Input: part model. Units: mm. Frame: model coordinates. A direction names the side the tool comes from. Coordinates: 2 decimals unless noted, no trailing zeros. Order: outer loops, then holes, each group sorted by start corner. A loop starts at its lowest first (then second) coordinate and runs counter-clockwise, first axis right, second up. Notation, with made-up numbers: M -28.75,32 L 20.25,32 A12 cw 20.25,54 Z; hole C 64,54 d4. An arc over 180 degrees is marked long. One line per item, written item: value.
```python
from build123d import *

# Parameters (mm, degrees)
BOSS_EXTRUDE1_DEPTH = 12.7
CUT_EXTRUDE2_DEPTH  = 199.932436772
CUT_EXTRUDE1_DEPTH  = 104.050150898
CUT_EXTRUDE3_DEPTH  = 63.5
CHAMFER1_SIZE       = 1.5875
FILLET1_R           = 0.762
FILLET2_R           = 1.27
CUT_EXTRUDE4_DEPTH  = 100.247182118


# Some blends are built 0.0001 mm under size
with BuildPart() as part:
    # Sketch1 → Boss-Extrude1 (new body)
    with BuildSketch(Plane(origin=(0, 0, 0), x_dir=(1, 0, 0), z_dir=(0, 1, 0))):
        with BuildLine():
            Line((-99.06, -12.7), (99.06, -12.7))
            Line((99.06, -12.7), (99.06, -11.1125))
            Line((99.06, -11.1125), (80.01, -11.1125))
            ThreePointArc((80.01, -11.1125), (75.519871939, -9.252628061), (73.66, -4.7625))
            Line((73.66, -4.7625), (73.66, 4.7625))
            ThreePointArc((73.66, 4.7625), (75.519871939, 9.252628061), (80.01, 11.1125))
            Line((80.01, 11.1125), (99.06, 11.1125))
            Line((99.06, 11.1125), (99.06, 12.7))
            Line((99.06, 12.7), (-99.06, 12.7))
            Line((-99.06, 12.7), (-99.06, 11.1125))
            Line((-99.06, 11.1125), (-80.01, 11.1125))
            ThreePointArc((-80.01, 11.1125), (-75.519871939, 9.252628061), (-73.66, 4.7625))
            Line((-73.66, 4.7625), (-73.66, -4.7625))
            ThreePointArc((-73.66, -4.7625), (-75.519871939, -9.252628061), (-80.01, -11.1125))
            Line((-80.01, -11.1125), (-99.06, -11.1125))
            Line((-99.06, -11.1125), (-99.06, -12.7))
        make_face()
    extrude(amount=BOSS_EXTRUDE1_DEPTH)

    # Sketch3 → Cut-Extrude2 (cut, through all)
    with BuildSketch(Plane.ZY.offset(99.06)):
        Polygon((11.1125, 12.7), (4.7625, 12.7), (-4.7625, 12.7), (-11.1125, 12.7), (-9.525, 6.35), (9.525, 6.35), align=None)
    extrude(amount=-CUT_EXTRUDE2_DEPTH, mode=Mode.SUBTRACT)

    # Sketch2 → Cut-Extrude1 (cut, through all)
    with BuildSketch(Plane.XY.offset(12.7)):
        Polygon((73.66, 12.7), (-73.66, 12.7), (-67.31, 6.35), (67.31, 6.35), align=None)
        with BuildLine():
            Line((97.263948776, 4.553948776), (92.71, 0))
            Line((92.71, 0), (99.06, 0))
            Line((99.06, 0), (99.06, 12.7))
            Line((99.06, 12.7), (92.71, 12.7))
            Line((92.71, 12.7), (97.263948776, 8.146051224))
            ThreePointArc((97.263948776, 8.146051224), (98.007897552, 6.35), (97.263948776, 4.553948776))
        make_face()
        with BuildLine():
            ThreePointArc((-97.263948776, 4.553948776), (-98.007897552, 6.35), (-97.263948776, 8.146051224))
            Line((-97.263948776, 8.146051224), (-92.71, 12.7))
            Line((-92.71, 12.7), (-99.06, 12.7))
            Line((-99.06, 12.7), (-99.06, 0))
            Line((-99.06, 0), (-92.71, 0))
            Line((-92.71, 0), (-97.263948776, 4.553948776))
        make_face()
    extrude(amount=-CUT_EXTRUDE1_DEPTH, mode=Mode.SUBTRACT)

    # Sketch4 → Revolve1 (revolve)
    with BuildSketch(Plane.ZY.offset(90.17)):
        with BuildLine():
            Line((12.7, 6.35), (12.7, 11.43))
            ThreePointArc((12.7, 11.43), (13.881381744, 9.01113492), (14.2875, 6.35))
            Line((14.2875, 6.35), (12.7, 6.35))
        make_face()
    revolve1 = revolve(axis=Axis((-90.17, 6.35, 0), (0, 0, 1)))

    # Mirror1: Revolve1 across plane
    add(revolve1.mirror(Plane.XY))

    # Sketch5 → Revolve2 (revolve)
    with BuildSketch(Plane(origin=(90.17, 0, 0), x_dir=(0, 0, -1), z_dir=(1, 0, 0))):
        with BuildLine():
            Line((11.1125, 6.35), (11.1125, 11.43))
            ThreePointArc((11.1125, 11.43), (9.931118256, 9.01113492), (9.525, 6.35))
            Line((9.525, 6.35), (11.1125, 6.35))
        make_face()
    revolve2 = revolve(axis=Axis((90.17, 6.35, 0), (0, 0, -1)))

    # Mirror2: Revolve2 across plane
    add(revolve2.mirror(Plane.XY))

    # Sketch6 → Cut-Extrude3 (cut, symmetric)
    with BuildSketch(Plane(origin=(0, 0, 0), x_dir=(0, 0, -1), z_dir=(1, 0, 0))):
        Polygon((-12.7, 0), (-11.1125, 0), (-12.7, 1.5875), align=None)
        Polygon((11.1125, 0), (12.7, 1.5875), (12.7, 0), align=None)
    extrude(amount=CUT_EXTRUDE3_DEPTH, both=True, mode=Mode.SUBTRACT)

    # Chamfer1
    chamfer1_edges = [part.edges().sort_by_distance(p)[0] for p in [
        (63.5, 0, 11.90625),
        (63.5, 0, -11.90625),
        (-63.5, 0, -11.90625),
        (-63.5, 0, 11.90625),
    ]]
    chamfer(chamfer1_edges, length=CHAMFER1_SIZE - 0.0001)  # a hair under: the kernel refuses the full size

    # Fillet1
    fillet1_edges = [part.edges().sort_by_distance(p)[0] for p in [
        (-98.007897552, 6.35, 12.7),
        (-92.71, 12.7, -11.90625),
        (-94.986974388, 10.423025612, -11.1125),
        (-94.986974388, 10.423025612, -12.7),
        (-94.986974388, 10.423025612, 11.1125),
        (-92.71, 12.7, 11.90625),
        (-94.986974388, 2.276974388, 12.7),
        (-98.007897552, 6.35, -11.1125),
        (-98.007897552, 6.35, 11.1125),
        (-94.986974388, 2.276974388, -11.1125),
        (-94.986974388, 2.276974388, 11.1125),
        (-98.007897552, 6.35, -12.7),
        (-94.986974388, 2.276974388, -12.7),
        (-94.986974388, 10.423025612, 12.7),
        (98.007897552, 6.35, 12.7),
        (92.71, 12.7, 11.90625),
        (92.71, 12.7, -11.90625),
        (94.986974388, 10.423025612, 12.7),
        (94.986974388, 2.276974388, 11.1125),
        (94.986974388, 2.276974388, -11.1125),
        (94.986974388, 2.276974388, -12.7),
        (98.007897552, 6.35, 11.1125),
        (94.986974388, 10.423025612, 11.1125),
        (94.986974388, 10.423025612, -11.1125),
        (98.007897552, 6.35, -12.7),
        (94.986974388, 10.423025612, -12.7),
        (94.986974388, 2.276974388, 12.7),
        (98.007897552, 6.35, -11.1125),
    ]]
    fillet(fillet1_edges, radius=FILLET1_R)

    # Fillet2
    # the kernel refuses this fillet: 1.27 mm, written as the material it takes off along each edge
    with BuildSketch(Plane(origin=(-75.90506403, 14.94506403, -12.7), x_dir=(-0.7071067811865446, -0.7071067811865505, 0), z_dir=(0.7071067811865506, -0.7071067811865446, 0))) as fillet2_piece_1_section:
        with BuildLine():
            CenterArc((FILLET2_R, -FILLET2_R), FILLET2_R, 90, 90)
            Line((0, -FILLET2_R), (0, 0))
            Line((0, 0), (FILLET2_R, 0))
        make_face()
    fillet2_piece_1 = extrude(amount=15.330256121, mode=Mode.PRIVATE)
    fillet2_piece_1 = split(fillet2_piece_1, bisect_by=Plane(origin=(-71.905795305, 6.35, -12.408746665), z_dir=(0, 1, 0)), keep=Keep.TOP, mode=Mode.PRIVATE)
    add(fillet2_piece_1, mode=Mode.SUBTRACT)
    with BuildSketch(Plane(origin=(-65.450815483, 4.490815483, -9.060203871), x_dir=(0.1230914909792504, -0.12309149097924957, -0.9847319278346824), z_dir=(-0.696310623822809, 0.6963106238228031, -0.17407765595558086))) as fillet2_piece_2_section:
        with BuildLine():
            CenterArc((FILLET2_R * 0.840960781889, FILLET2_R), FILLET2_R, 189.874961398, 80.125038602)
            Line((-FILLET2_R * 0.144223584254, FILLET2_R * 0.828501414858), (0, 0))
            Line((0, 0), (FILLET2_R * 0.840960781889, 0))
        make_face()
    fillet2_piece_2 = extrude(amount=14.459594166, mode=Mode.PRIVATE)
    fillet2_piece_2 = split(fillet2_piece_2, bisect_by=Plane(origin=(-71.646234354, 6.35, -10.770930609), z_dir=(0, 1, 0)), keep=Keep.TOP, mode=Mode.PRIVATE)
    add(fillet2_piece_2, mode=Mode.SUBTRACT)
    with BuildSketch(Plane(origin=(-75.519184517, 14.559184517, 11.577296129), x_dir=(-0.7177405625652845, -0.6755205294731655, -0.1688801323683837), z_dir=(0.69631062382278, -0.6963106238227741, -0.17407765595581334))) as fillet2_piece_3_section:
        with BuildLine():
            CenterArc((FILLET2_R * 0.840960781889, -FILLET2_R), FILLET2_R, 90, 80.125038602)
            Line((-FILLET2_R * 0.144223584254, -FILLET2_R * 0.828501414857), (0, 0))
            Line((0, 0), (FILLET2_R * 0.840960781889, 0))
        make_face()
    fillet2_piece_3 = extrude(amount=14.459594166, mode=Mode.PRIVATE)
    fillet2_piece_3 = split(fillet2_piece_3, bisect_by=Plane(origin=(-71.646234354, 6.35, 10.770930609), z_dir=(0, 1, 0)), keep=Keep.TOP, mode=Mode.PRIVATE)
    add(fillet2_piece_3, mode=Mode.SUBTRACT)
    with BuildSketch(Plane(origin=(-75.90506403, 14.94506403, 12.7), x_dir=(-0.7071067811865445, -0.7071067811865505, 0), z_dir=(0.7071067811865506, -0.7071067811865446, 0))) as fillet2_piece_4_section:
        with BuildLine():
            CenterArc((FILLET2_R, FILLET2_R), FILLET2_R, 180, 90)
            Line((0, FILLET2_R), (0, 0))
            Line((0, 0), (FILLET2_R, 0))
        make_face()
    fillet2_piece_4 = extrude(amount=15.330256121, mode=Mode.PRIVATE)
    fillet2_piece_4 = split(fillet2_piece_4, bisect_by=Plane(origin=(-71.905795305, 6.35, 12.408746665), z_dir=(0, 1, 0)), keep=Keep.TOP, mode=Mode.PRIVATE)
    add(fillet2_piece_4, mode=Mode.SUBTRACT)
    with BuildSketch(Plane(origin=(65.06493597, 4.10493597, -12.7), x_dir=(0.7071067811865445, -0.7071067811865506, 0), z_dir=(0.7071067811865506, 0.7071067811865445, 0))) as fillet2_piece_5_section:
        with BuildLine():
            CenterArc((FILLET2_R, -FILLET2_R), FILLET2_R, 90, 90)
            Line((0, -FILLET2_R), (0, 0))
            Line((0, 0), (FILLET2_R, 0))
        make_face()
    fillet2_piece_5 = extrude(amount=15.330256121, mode=Mode.PRIVATE)
    fillet2_piece_5 = split(fillet2_piece_5, bisect_by=Plane(origin=(71.905795305, 6.35, -12.408746665), z_dir=(0, 1, 0)), keep=Keep.TOP, mode=Mode.PRIVATE)
    add(fillet2_piece_5, mode=Mode.SUBTRACT)
    with BuildSketch(Plane(origin=(75.519184517, 14.559184517, -11.577296129), x_dir=(-0.12309149097927001, -0.12309149097926336, -0.9847319278346782), z_dir=(-0.6963106238228061, -0.6963106238228001, 0.17407765595560445))) as fillet2_piece_6_section:
        with BuildLine():
            CenterArc((FILLET2_R * 0.840960781889, FILLET2_R), FILLET2_R, 189.874961398, 80.125038602)
            Line((-FILLET2_R * 0.144223584254, FILLET2_R * 0.828501414858), (0, 0))
            Line((0, 0), (FILLET2_R * 0.84096078189, 0))
        make_face()
    fillet2_piece_6 = extrude(amount=14.459594166, mode=Mode.PRIVATE)
    fillet2_piece_6 = split(fillet2_piece_6, bisect_by=Plane(origin=(71.646234354, 6.35, -10.770930609), z_dir=(0, 1, 0)), keep=Keep.TOP, mode=Mode.PRIVATE)
    add(fillet2_piece_6, mode=Mode.SUBTRACT)
    with BuildSketch(Plane(origin=(65.06493597, 4.10493597, 12.7), x_dir=(0.7071067811865445, -0.7071067811865507, 0), z_dir=(0.7071067811865506, 0.7071067811865445, 0))) as fillet2_piece_7_section:
        with BuildLine():
            CenterArc((FILLET2_R, FILLET2_R), FILLET2_R, 180, 90)
            Line((0, FILLET2_R), (0, 0))
            Line((0, 0), (FILLET2_R, 0))
        make_face()
    fillet2_piece_7 = extrude(amount=15.330256121, mode=Mode.PRIVATE)
    fillet2_piece_7 = split(fillet2_piece_7, bisect_by=Plane(origin=(71.905795305, 6.35, 12.408746665), z_dir=(0, 1, 0)), keep=Keep.TOP, mode=Mode.PRIVATE)
    add(fillet2_piece_7, mode=Mode.SUBTRACT)
    with BuildSketch(Plane(origin=(65.450815483, 4.490815483, 9.060203871), x_dir=(0.7177405625652817, -0.6755205294731627, -0.16888013236840813), z_dir=(0.6963106238227829, 0.6963106238227769, 0.1740776559557897))) as fillet2_piece_8_section:
        with BuildLine():
            CenterArc((FILLET2_R * 0.840960781889, -FILLET2_R), FILLET2_R, 90, 80.125038602)
            Line((-FILLET2_R * 0.144223584254, -FILLET2_R * 0.828501414857), (0, 0))
            Line((0, 0), (FILLET2_R * 0.840960781889, 0))
        make_face()
    fillet2_piece_8 = extrude(amount=14.459594166, mode=Mode.PRIVATE)
    fillet2_piece_8 = split(fillet2_piece_8, bisect_by=Plane(origin=(71.646234354, 6.35, 10.770930609), z_dir=(0, 1, 0)), keep=Keep.TOP, mode=Mode.PRIVATE)
    add(fillet2_piece_8, mode=Mode.SUBTRACT)

    # Sketch7 → Cut-Extrude4 (cut, through all)
    with BuildSketch(Plane(origin=(0, 6.35, 0), x_dir=(1, 0, 0), z_dir=(0, 1, 0))):
        with BuildLine():
            Line((-22.86, 9.525), (62.23, 9.525))
            ThreePointArc((62.23, 9.525), (65.822102448, 8.037102448), (67.31, 4.445))
            Line((67.31, 4.445), (67.31, -4.445))
            ThreePointArc((67.31, -4.445), (65.822102448, -8.037102448), (62.23, -9.525))
            Line((62.23, -9.525), (-22.86, -9.525))
            ThreePointArc((-22.86, -9.525), (-26.452102448, -8.037102448), (-27.94, -4.445))
            Line((-27.94, -4.445), (-27.94, 4.445))
            ThreePointArc((-27.94, 4.445), (-26.452102448, 8.037102448), (-22.86, 9.525))
        make_face()
    extrude(amount=-CUT_EXTRUDE4_DEPTH, mode=Mode.SUBTRACT)


solid = part.part
```
(1) First-contact query: pin 1 (2 mm diameter, centred on x = -75, y = 4, fed in from +Z); pin 2 (4 mm diameter, centred on x = -13.5, y = 2.5, fed in from -Z); pin 3 (3 mm diameter, centred on y = 4, z = -0.5, fed in from +X); pin 4 (2 mm diameter, centred on x = -73, z = 8, fed in from -Y). Flat tips, straight axial feed; report the tip coordinate or a pass-through.
Data:
pin 1: stops at z = 12.7
pin 2: stops at z = -12.7
pin 3: stops at x = 73.66
pin 4: stops at y = 0
(2) Cut plane B-B on z = -2. Output: boundary loops of the cut face in (x, y), plus the area to 3 significant figures.
Data:
outline: M -73.66,0 L -27.94,0 L -27.94,6.35 L -73.66,6.35 Z; M 67.31,0 L 73.66,0 L 73.66,6.35 L 67.31,6.35 Z
area: 331 mm2
(3) Access query for faces 5 (the flat face through (84.9, 6.3, 11.112)), 6 (the cylindrical face through (-94.591, 2.205, 11.33)), 7 (the cylindrical face through (-71.131, 9.739, 10.671)). Directions: +Z, -Z, +X, -X, +Y, -Y. A direction counts if a zero-diameter tool reaches every point of the face in a straight line with its end or side. Return the directions, or none.
Data:
face 5: none
face 6: -X, -Y
face 7: +Y
(4) Ray query, line 1 (Z direction, x = -3.5, y = 2) (3 decimals); line 2 (X direction, y = 5.25, z = -0.5); line 3 (Z direction, x = 87, y = 10.5). Return the intervals inside material, ascending. Write a range as from..to.
Data:
line 1: z = -12.7..-9.525, 9.525..12.7
line 2: x = -73.66..-27.94, 67.31..73.66
line 3: z = -12.7..-11.11, 11.11..12.7
(5) Draft query along X for faces 1 (the cylindrical face through (-71.25, 9.75, -12.34)), 2 (the cylindrical face through (94.52, 2.13, 12.48)), 3 (the cylindrical face through (-94.52, 10.57, 12.48)), 4 (the flat face through (-74.482, 8.864, -10.153)). Return one class per face: released by +X, released by -X, zero draft, split by the parting line, or undercut.
Data:
face 1: undercut
face 2: released by +X
face 3: released by -X
face 4: zero draft
